Can you work these out from the model? Positions are in its coordinate system, mm. A direction names the side the tool comes from. Round coordinates to 2 decimals unless told otherwise and drop trailing zeros. Loops run counter-clockwise (first coordinate to the right, second up) from the corner with the lowest first, then second, coordinate; pieces in that order, holes last. Notation, with made-up numbers: (56.25, 47) -> (69.25, 47) arc R21 cw to (69.25, 78) -> close; hole circle Ø3 at (-7.5, 52). An arc over 180 degrees is marked (long way). Write each question's results on one line, items separated by ' | '.
from build123d import *

# Parameters (mm, degrees)
F0_W      = 139.446
F0_H      = 14.999996
F1_DEPTH  = 38.1
F2_W      = 139.446
F2_H      = 19.567398
F3_DEPTH  = 8.000009
F5_W      = 12.7
F5_H      = 12.7
F6_DEPTH  = 21.844
F9_R      = 1.730591
F10_DEPTH = 42.164
F12_W     = 50.999898
F12_H     = 50.999898
F13_DEPTH = 1.5
F14_DEPTH = 12.000001


with BuildPart() as f1:
    # F0 (on Front) → F1 (new body, symmetric)
    with BuildSketch(Plane.XZ):
        Rectangle(F0_W, F0_H)
    extrude(amount=F1_DEPTH, both=True)

    # F2 (on face) → F3 (cut)
    with BuildSketch(Plane.XY.offset(7.499998)):
        with Locations((0, -28.316301)):
            Rectangle(F2_W, F2_H)
    extrude(amount=-F3_DEPTH, mode=Mode.SUBTRACT)

    # F4: F1 across plane


with BuildPart() as f1_1:
    add(f1.part)
    add(f1.part.mirror(Plane.XZ), mode=Mode.INTERSECT)

    # F5 (on face) → F6 (cut)
    with BuildSketch(Plane.XY.offset(7.499998)):
        with Locations((59.793662, -9.017324)):
            Rectangle(F5_W, F5_H)
    extrude(amount=-F6_DEPTH, mode=Mode.SUBTRACT)

    # F7: F1 across plane


with BuildPart() as f1_2:
    add(f1_1.part)
    add(f1_1.part.mirror(Plane.XZ), mode=Mode.INTERSECT)

    # F8: F1 across plane


with BuildPart() as f1_3:
    add(f1_2.part)
    add(f1_2.part.mirror(Plane.YZ), mode=Mode.INTERSECT)

    # F9 (on Top) → F10 (cut)
    with BuildSketch(Plane.XY):
        with Locations((53.080564, -23.971872)):
            Circle(F9_R)
        with Locations((53.080564, 23.971872)):
            Circle(F9_R)
        with Locations((-53.080564, 23.971872)):
            Circle(F9_R)
        with Locations((-53.080564, -23.971872)):
            Circle(F9_R)
    extrude(amount=-F10_DEPTH, mode=Mode.SUBTRACT)

    # F12 (on face) → F13 (cut)
    with BuildSketch(Plane(origin=(0, 0, -7.499998), x_dir=(1, 0, 0), z_dir=(0, 0, -1))):
        Rectangle(F12_W, F12_H)
    extrude(amount=-F13_DEPTH, mode=Mode.SUBTRACT)

    # F11 (on face) → F14 (cut)
    with BuildSketch(Plane(origin=(0, 0, -7.499998), x_dir=(1, 0, 0), z_dir=(0, 0, -1))):
        Polygon((69.723, -13.90828), (69.723, 14.091664), (1.722882, 14.091664), (-69.723, 14.091664), (-69.723, -13.90828), (1.722882, -13.90828), align=None)
    extrude(amount=-F14_DEPTH, mode=Mode.SUBTRACT)


solid = f1_3.part
1. Please list where these lines run through material, in increasing order: line 1 (X direction, y = -15, z = -3); line 2 (Y direction, x = 30, z = -1.25); line 3 (Y direction, x = 30, z = 3.75). Write a range as from..to.
Final values:
line 1: -69.72..-66.14, -53.44..53.44, 66.14..69.72 | line 2: -38.1..-14.09, 13.91..38.1 | line 3: -18.53..-14.09, 13.91..18.53
2. If we section it at C-C (y = 12): List the corners of the cut face in (x, z) for me.
Final values:
outline: (-69.72, 4.5) -> (-66.14, 4.5) -> (-66.14, 7.5) -> (-69.72, 7.5) -> close; (-53.44, 4.5) -> (53.44, 4.5) -> (53.44, 7.5) -> (-53.44, 7.5) -> close; (66.14, 4.5) -> (69.72, 4.5) -> (69.72, 7.5) -> (66.14, 7.5) -> close
3. If we section it at D-D (x = 19): List the corners of the cut face in (y, z) for me.
Final values:
outline: (-38.1, -7.5) -> (-25.5, -7.5) -> (-25.5, -6) -> (-14.09, -6) -> (-14.09, 4.5) -> (13.91, 4.5) -> (13.91, -6) -> (25.5, -6) -> (25.5, -7.5) -> (38.1, -7.5) -> (38.1, -0.5) -> (18.53, -0.5) -> (18.53, 7.5) -> (-18.53, 7.5) -> (-18.53, -0.5) -> (-38.1, -0.5) -> close
4. If we section it at A-A (x = 60): List the corners of the cut face in (y, z) for me.
Final values:
outline: (-38.1, -7.5) -> (-15.37, -7.5) -> (-15.37, 7.5) -> (-18.53, 7.5) -> (-18.53, -0.5) -> (-38.1, -0.5) -> close; (-2.67, 4.5) -> (2.67, 4.5) -> (2.67, 7.5) -> (-2.67, 7.5) -> close; (15.37, -7.5) -> (38.1, -7.5) -> (38.1, -0.5) -> (18.53, -0.5) -> (18.53, 7.5) -> (15.37, 7.5) -> close
5. Will these pins go through, and if not, where does the flat tip stop? pin 1 (1.5 mm diameter, centred on x = -57, z = 6, fed in from +Y); pin 2 (3.5 mm diameter, centred on x = 7, y = -20, fed in from -Z); pin 3 (10 mm diameter, centred on x = -1.5, y = -27.5, fed in from +Z); pin 4 (4 mm diameter, centred on y = -10.5, z = -2, fed in from +X).
Final values:
pin 1: y = 18.53 | pin 2: z = -6 | pin 3: z = -0.5 | pin 4: through
6. We'd pull the mould along Y, two halves only. Please class faces 4 (the face through (-1, 29, -7.5)), 5 (the face through (0, -20, -6)), 6 (the face through (-1, -18.533, 4)): pulls with the +Y half, pulls with the -Y half, needs draft (parallel to the pull), parting line crosses it, or undercut.
Final values:
face 4: needs draft | face 5: undercut | face 6: pulls with the -Y half
7. If we section it at B-B (z = -3.5): List the corners of the cut face in (x, y) for me.
Final values:
outline: (-69.72, -38.1) -> (69.72, -38.1) -> (69.72, -14.09) -> (66.14, -14.09) -> (66.14, -15.37) -> (53.44, -15.37) -> (53.44, -14.09) -> (-53.44, -14.09) -> (-53.44, -15.37) -> (-66.14, -15.37) -> (-66.14, -14.09) -> (-69.72, -14.09) -> close; (-69.72, 13.91) -> (-66.14, 13.91) -> (-66.14, 15.37) -> (-53.44, 15.37) -> (-53.44, 13.91) -> (53.44, 13.91) -> (53.44, 15.37) -> (66.14, 15.37) -> (66.14, 13.91) -> (69.72, 13.91) -> (69.72, 38.1) -> (-69.72, 38.1) -> close; hole circle Ø3.46 at (-53.08, -23.97); hole circle Ø3.46 at (-53.08, 23.97); hole circle Ø3.46 at (53.08, -23.97); hole circle Ø3.46 at (53.08, 23.97)
8. On a 3-axis mill with a long thin cutter (end or side, diameter ignored), from which of +Z, -Z, +X, -X, +Y, -Y can I reach the whole of each face in a straight line? I mean faces 1 (the face through (-1, 0, 4.5)), 2 (the face through (-60, -2.667, 6)), 3 (the face through (-1, 0, 7.5)). Say none if no direction works.
Final values:
face 1: -Z, +X, -X | face 2: +Z, -Z | face 3: +Z, +X, -X, +Y, -Y
